from build123d import *

# Parameters (mm, degrees)
SKETCH1_W           = 66.04
SKETCH1_H           = 10.16
BOSS_EXTRUDE1_DEPTH = 66.04
SKETCH5_W           = 66.04
SKETCH5_H           = 57.15
BOSS_EXTRUDE2_DEPTH = 30.48
SKETCH6_W           = 38.1
SKETCH6_H           = 30.48
CUT_EXTRUDE4_DEPTH  = 67.04
SKETCH7_R           = 1.27
CUT_EXTRUDE5_DEPTH  = 7.62
BOSS_EXTRUDE3_DEPTH = 66.04
FILLET1_R           = 1.27
SKETCH9_R           = 2.54
CUT_EXTRUDE6_DEPTH  = 10.16


with BuildPart() as part:
    # Sketch1 → Boss-Extrude1 (new body)
    with BuildSketch(Plane.XY):
        with Locations((33.02, 5.08)):
            Rectangle(SKETCH1_W, SKETCH1_H)
    extrude(amount=BOSS_EXTRUDE1_DEPTH)

    # Sketch5 → Boss-Extrude2 (add)
    with BuildSketch(Plane(origin=(0, 10.16, 0), x_dir=(1, 0, 0), z_dir=(0, 1, 0))):
        with Locations((33.02, -33.02)):
            Rectangle(SKETCH5_W, SKETCH5_H)
    extrude(amount=BOSS_EXTRUDE2_DEPTH)

    # Sketch6 → Cut-Extrude4 (cut, through all)
    with BuildSketch(Plane.ZY):
        with Locations((33.02, 15.24)):
            Rectangle(SKETCH6_W, SKETCH6_H)
    extrude(amount=-CUT_EXTRUDE4_DEPTH, mode=Mode.SUBTRACT)

    # Sketch7 → Cut-Extrude5 (cut)
    with BuildSketch(Plane(origin=(0, 40.64, 0), x_dir=(1, 0, 0), z_dir=(0, 1, 0))):
        with Locations((6.985, -57.15)):
            Circle(SKETCH7_R)
        with Locations((8.255, -8.89)):
            Circle(SKETCH7_R)
        with Locations((59.055, -24.13)):
            Circle(SKETCH7_R)
        with Locations((59.055, -52.07)):
            Circle(SKETCH7_R)
        with Locations((43.18, -38.608)):
            Circle(SKETCH7_R)
        with Locations((22.86, -38.608)):
            Circle(SKETCH7_R)
    extrude(amount=-CUT_EXTRUDE5_DEPTH, mode=Mode.SUBTRACT)

    # Sketch8 → Boss-Extrude3 (add)
    with BuildSketch(Plane(origin=(66.04, 0, 0), x_dir=(0, 0, -1), z_dir=(1, 0, 0))):
        Polygon((-61.595, 10.16), (-66.04, 10.16), (-61.595, 40.64), align=None)
        Polygon((-4.445, 10.16), (-4.445, 40.64), (0, 10.16), align=None)
    extrude(amount=-BOSS_EXTRUDE3_DEPTH)

    # Fillet1
    fillet1_edges = [part.edges().sort_by_distance(p)[0] for p in [
        (66.04, 5.08, 66.04),
        (33.02, 0, 66.04),
        (66.04, 0, 6.985),
        (66.04, 15.24, 52.07),
        (66.04, 30.48, 33.02),
        (66.04, 15.24, 13.97),
        (0, 0, 6.985),
        (33.02, 0, 52.07),
        (33.02, 0, 13.97),
        (0, 15.24, 13.97),
        (33.02, 30.48, 13.97),
        (0, 30.48, 33.02),
        (33.02, 30.48, 52.07),
        (0, 15.24, 52.07),
        (0, 5.08, 66.04),
        (33.02, 0, 0),
        (66.04, 5.08, 0),
        (33.02, 10.16, 0),
        (0, 5.08, 0),
        (33.02, 10.16, 66.04),
        (66.04, 25.4, 63.8175),
        (0, 25.4, 63.8175),
        (0, 0, 59.055),
        (66.04, 0, 59.055),
        (66.04, 25.4, 2.2225),
        (0, 25.4, 2.2225),
    ]]
    fillet(fillet1_edges, radius=FILLET1_R)

    # Sketch9 → Cut-Extrude6 (cut)
    with BuildSketch(Plane.XZ):
        with Locations((58.42, 58.42)):
            Circle(SKETCH9_R)
        with Locations((7.62, 58.42)):
            Circle(SKETCH9_R)
        with Locations((7.62, 7.62)):
            Circle(SKETCH9_R)
        with Locations((58.42, 7.62)):
            Circle(SKETCH9_R)
    extrude(amount=-CUT_EXTRUDE6_DEPTH, mode=Mode.SUBTRACT)


solid = part.part
Part model, mm, in its own coordinate system. A direction names the side the tool comes from. Round coordinates to 2 decimals unless told otherwise and drop trailing zeros. Write each loop counter-clockwise with the first axis right and the second up, starting at its lowest first coordinate (ties: lowest second). Pieces come first, ordered by that corner, then holes. Notation, with made-up numbers: M 72,82 L 98,82 A9 cw 98,94 Z; hole C 83.5,-26.5 d3. An arc over 180 degrees is marked long. Return JSON: item names as keys, results as strings. Group by question number.
(1) Saw through at B-B on x = 43.18. Write the cut outline in (y, z) (3 decimals), then the cut area to 3 significant figures.
(2) Which spindle directions (+Z, -Z, +X, -X, +Y, -Y) get a long thin tool onto all of the face, cutting with end or side? Do faces 1 (the face through (7.07, 5.01, 5.14)), 2 (the face through (33, 15, 52.07)), 3 (the face through (43, 33.02, 39)). Say none if no direction does.
(3) Drill centre lines: probe 1 along X at (y, z) = (35, 52); probe 2 along Y at (x, z) = (45, 29); probe 3 along Z at (x, y) = (31, 8). Where is each one in solid material? Low to high.
(4) Pin check, flat tips, straight feed: pin 1 Ø3 at (x, z) = (7.62, 58.42) entering from -Y; pin 2 Ø8.5 at (x, y) = (21, 19) entering from +Z; pin 3 Ø8 at (x, y) = (49.5, 14.5) entering from +Z. Stop position of each tip, or through.
(5) Saw through at C-C on z = 19. Write the cut outline in (x, y).
(6) Saw through at A-A on y = 8. Write the cut outline in (x, z), then the cut area to 3 significant figures.
(7) Saw through at D-D on z = 8.89. Write the cut outline in (x, y) (3 decimals), then the cut area to 3 significant figures.
Returned:
{
 "1": {"outline": "M 0,1.27 A1.27 ccw 1.27,0 L 10.068,0 A1.27 ccw 10.251,0.013 L 40.64,4.445 L 40.64,37.338 L 33.02,37.338 L 33.02,39.878 L 40.64,39.878 L 40.64,61.595 L 10.251,66.027 A1.27 ccw 10.068,66.04 L 1.27,66.04 A1.27 ccw 0,64.77 L 0,53.34 A1.27 ccw 1.27,52.07 L 29.21,52.07 A1.27 cw 30.48,50.8 L 30.48,15.24 A1.27 cw 29.21,13.97 L 1.27,13.97 A1.27 ccw 0,12.7 Z", "area": "1,370 mm²"},
 "2": {"face 1": "-Y", "face 2": "+X, -X, -Y", "face 3": "+Y"},
 "3": {"probe 1": "0 to 57.79, 60.32 to 66.04", "probe 2": "30.48 to 40.64", "probe 3": "0 to 13.97, 52.07 to 66.04"},
 "4": {"pin 1": "y = 10.16", "pin 2": "z = 65.37", "pin 3": "z = 65.99"},
 "5": {"outline": "M 0,31.75 A1.27 ccw 1.27,30.48 L 64.77,30.48 A1.27 ccw 66.04,31.75 L 66.04,40.64 L 0,40.64 Z"},
 "6": {"outline": "M 0,1.27 A1.27 ccw 1.27,0 L 64.77,0 A1.27 ccw 66.04,1.27 L 66.04,12.7 A1.27 ccw 64.77,13.97 L 1.27,13.97 A1.27 ccw 0,12.7 Z; M 0,53.34 A1.27 ccw 1.27,52.07 L 64.77,52.07 A1.27 ccw 66.04,53.34 L 66.04,64.77 A1.27 ccw 64.77,66.04 L 1.27,66.04 A1.27 ccw 0,64.77 Z; hole C 7.62,7.62 d5.08; hole C 7.62,58.42 d5.08; hole C 58.42,7.62 d5.08; hole C 58.42,58.42 d5.08", "area": "1,760 mm²"},
 "7": {"outline": "M 0,1.27 A1.27 ccw 1.27,0 L 5.42,0 L 5.42,10.16 L 9.82,10.16 L 9.82,0 L 56.22,0 L 56.22,10.16 L 60.62,10.16 L 60.62,0 L 64.77,0 A1.27 ccw 66.04,1.27 L 66.04,40.64 L 9.525,40.64 L 9.525,33.02 L 6.985,33.02 L 6.985,40.64 L 0,40.64 Z", "area": "2,570 mm²"}
}
